```python
from build123d import *

# Parameters (mm, degrees)
SKETCH2_R           = 5.08
BOSS_EXTRUDE2_DEPTH = 41.91
SKETCH3_W           = 8.89
SKETCH3_H           = 6.35


with BuildPart() as part:
    # Sketch2 → Boss-Extrude2 (new body)
    with BuildSketch(Plane(origin=(0, 0, 0), x_dir=(-1, 0, 0), z_dir=(0, 1, 0))):
        with Locations(Location((0, 0, 0), (0, 0, 90))):
            Circle(SKETCH2_R)
    extrude(amount=BOSS_EXTRUDE2_DEPTH)

    # Sketch3 → Revolve1 (revolve)
    with BuildSketch(Plane.XY, mode=Mode.PRIVATE) as revolve1_sk:
        with Locations((-4.445, 10.795)):
            Rectangle(SKETCH3_W, SKETCH3_H)
    revolve(revolve1_sk.sketch.rotate(Axis((0, 0, 0), (0, 1, 0)), 270), axis=Axis((0, 0, 0), (0, 1, 0)))

    # Sketch4 → Revolve2 (revolve)
    with BuildSketch(Plane(origin=(0, 41.91, 0), x_dir=(1, 0, 0), z_dir=(0, 1, 0)), mode=Mode.PRIVATE) as revolve2_sk:
        with BuildLine():
            Line((0, 5.08), (-65.278, 5.08))
            Line((-65.278, 5.08), (-65.278, 0))
            Line((-65.278, 0), (5.08, 0))
            ThreePointArc((5.08, 0), (3.592102448, 3.592102448), (0, 5.08))
        make_face()
    revolve(revolve2_sk.sketch.rotate(Axis((-65.278, 41.91, 0), (1, 0, 0)), 180), axis=Axis((-65.278, 41.91, 0), (1, 0, 0)))

    # Sketch5 → Revolve3 (revolve)
    with BuildSketch(Plane.ZY.offset(65.278), mode=Mode.PRIVATE) as revolve3_sk:
        with BuildLine():
            Line((0, 46.99), (0, 24.13))
            Line((0, 24.13), (-5.08, 24.13))
            Line((-5.08, 24.13), (-5.08, 41.91))
            ThreePointArc((-5.08, 41.91), (-3.592102448, 45.502102448), (0, 46.99))
        make_face()
    revolve(revolve3_sk.sketch.rotate(Axis((-65.278, 46.99, 0), (0, -1, 0)), 180), axis=Axis((-65.278, 46.99, 0), (0, -1, 0)))


solid = part.part
```
Geometry: final body of the model. Coordinates: model frame, mm. A direction names the side the tool comes from. Round coordinates to 2 decimals unless told otherwise and drop trailing zeros. Loops run counter-clockwise (first coordinate to the right, second up) from the corner with the lowest first, then second, coordinate; pieces in that order, holes last.
Item 1: Reachability of faces 4 (the flat face through (0, 0, 0)), 5 (the flat face through (4, 7.62, -4)), 6 (the cylindrical face through (-33.1, 46.87, -1.1)) from +Z, -Z, +X, -X, +Y, -Y: full face, straight path, thin tool, end or side. Return the list, or none.
Checked values:
face 4: +Z, -Z, +X, -X, -Y
face 5: -Y
face 6: none
Item 2: Section C-C, the plane y = 33.5. Output: boundary loops of the cut face in (x, z), plus the area to 3 significant figures.
Checked values:
outline: circle Ø10.16 at (-65.28, 0); circle Ø10.16 at (0, 0)
area: 162 mm2
Item 3: Line query: L1, parallel to Y at x = -1, z = -6.25; L2, parallel to Z at x = -36, y = 45; L3, parallel to X at y = 17, z = -3.75. Output: solid intervals per line, ascending.
Checked values:
L1: y = 7.62 to 13.97
L2: z = -4.03 to 4.03
L3: x = -3.43 to 3.43
Item 4: Contact query for flat-ended pins moving along their axis: P1, Ø5, axis at x = -67, z = 1.5, coming from the -Y side; P2, Ø10, axis at y = 13.5, z = -5.5, coming from the +X side; P3, Ø6, axis at y = 6.5, z = -5.5, coming from the -X side. Output: stop coordinate, or through.
Checked values:
P1: stops at y = 24.13
P2: stops at x = 8.88
P3: stops at x = -8.46
Item 5: Section D-D, the plane x = -34. Output: boundary loops of the cut face in (y, z).
Checked values:
outline: circle Ø10.16 at (41.91, 0)
Item 6: Mould query, pull axis Y, two halves, no side actions, for faces 1 (the cylindrical face through (8.68, 10.84, 1.93)), 2 (the flat face through (4, 13.97, -4)), 3 (the flat face through (-65, 24.13, 0)). Classes: released by +Y, released by -Y, zero draft, split by the parting line, or undercut.
Checked values:
face 1: zero draft
face 2: undercut
face 3: released by -Y
Item 7: Section B-B, the plane x = -8. Output: boundary loops of the cut face in (y, z), plus the area to 3 significant figures.
Checked values:
outline: (7.62, -3.88) - (13.97, -3.88) - (13.97, 3.88) - (7.62, 3.88) - close; circle Ø10.16 at (41.91, 0)
area: 130 mm2
Item 8: Section A-A, the plane z = 0. Output: boundary loops of the cut face in (x, y).
Checked values:
outline: (-70.36, 24.13) - (-60.2, 24.13) - (-60.2, 36.83) - (-5.08, 36.83) - (-5.08, 13.97) - (-8.89, 13.97) - (-8.89, 7.62) - (-5.08, 7.62) - (-5.08, 0) - (5.08, 0) - (5.08, 7.62) - (8.89, 7.62) - (8.89, 13.97) - (5.08, 13.97) - (5.08, 41.91) arc R5.08 ccw to (0, 46.99) - (-65.28, 46.99) arc R5.08 ccw to (-70.36, 41.91) - close
